For this review, take the finished solid that the model builds, in its own axes (mm). Give positions to 0.01 mm unless a question says otherwise; leave off trailing zeros. Order: outer loops, then holes, each group sorted by start corner. A loop starts at its lowest first (then second) coordinate and runs counter-clockwise, first axis right, second up. Notation, with made-up numbers: (-4.5, 31.5) -> (32.5, 31.5) arc R15 ccw to (32.5, 45.5) -> close; hole circle Ø7 at (68, 6). An arc over 180 degrees is marked (long way). Use CSV: the item, a comma, the result in double quotes. Start each with the question number.
Autodesk Inventor part; units mm, degrees
ref_plane "YZ Plane" through (0, 0, 0) normal (1, 0, 0) x (0, 1, 0)
ref_plane "XZ Plane" through (0, 0, 0) normal (0, 1, 0) x (-1, 0, 0)
ref_plane "XY Plane" through (0, 0, 0) normal (0, 0, 1) x (1, 0, 0)
sketch "Sketch1" plane through (0, 0, 0) normal (0, 1, 0) x (-1, 0, 0)
  line L0 (0, 0) -> (20.2618, 0)
  line L1 (20.2618, 0) -> (20.2618, -15.5601)
  line L2 (20.2618, -15.5601) -> (0, -15.5601)
  line L3 (0, -15.5601) -> (0, 0)
  dimension "d0" = 20.2618
  dimension "d1" = 15.5601
extrude "Extrusion1" add sketch "Sketch1" along normal blind 2.54
sketch "Sketch2" plane through (0, 2.54, 0) normal (0, 1, 0) x (1, 0, 0)
  circle A0 centre (-19.0703, 1.3447) radius 0.8937
  line L0 (-20.2618, 15.5601) -> (-20.2618, 0) construction
  line L1 (-20.2618, 0) -> (0, 0) construction
  line L2 (-20.2618, 0) -> (0, 0) construction
  circle A1 centre (-16.5303, 1.3447) radius 0.8937
  circle A2 centre (-13.9903, 1.3447) radius 0.8937
  circle A3 centre (-11.4503, 1.3447) radius 0.8937
  circle A4 centre (-8.9103, 1.3447) radius 0.8937
  circle A5 centre (-6.3703, 1.3447) radius 0.8937
  circle A6 centre (-3.8303, 1.3447) radius 0.8937
  circle A7 centre (-1.2903, 1.3447) radius 0.8937
  circle A8 centre (-17.7809, 13.0792) radius 1.5
  circle A9 centre (-2.4809, 13.0792) radius 1.5
  line L3 (0, 15.5601) -> (-20.2618, 15.5601)
  line L4 (0, 0) -> (0, 15.5601)
  line L5 (-17.7809, 13.0792) -> (-2.4809, 13.0792) construction
  line L6 (-10.1309, 0) -> (-10.1309, 15.5601) construction
  point P0 (-10.1309, 13.0792)
  dimension "d6" = 2.54
  dimension "d11" = 3
  dimension "d12" = 3
  dimension "d17" = 15.3
  dimension "d18" = 2.4809
  dimension "d19" = 2.4809
extrude "Extrusion2" cut sketch "Sketch2" against normal up to next
sketch "Sketch3" plane through (0, 2.54, 0) normal (0, 1, 0) x (1, 0, 0)
  line L0 (-14.6694, 9.1277) -> (-2.5672, 9.1277) construction
  line L1 (-2.5672, 9.1277) -> (-2.5672, 4.9306) construction
  line L2 (-2.5672, 4.9306) -> (-14.6694, 4.9306) construction
  line L3 (-14.6694, 4.9306) -> (-14.6694, 9.1277) construction
  point P0 (0, 0)
equation "\"d19\" = d18"
properties part number "IMU_temp"
1. Consider section C-C (z = -13.5). State the section outline as (x, y) points.
2. Consider section A-A (x = -9). State the section outline as (y, z) points, plus the area to 3 significant figures.
3. Consider section B-B (y = 0.4). State how many separate pieces and enclosed holes the cut face has, plus the area to 3 significant figures.
4. Draft analysis for pull direction X (two halves, no side actions). For faces 1 (the face through (-20.262, 1, -8)), 2 (the face through (0, 1, -8)), 3 (the face through (-10, 1, -15.56)), 4 (the face through (-15.705, 1.288, -1.002)), state which applies: +X half, -X half, draft (parallel to the pull), parting line (faces both ways), or undercut.
5. To check wall thickness, follow L1, parallel to X at y = 0.5, z = -13; L2, parallel to Z at x = -1.75, y = 0.65; L3, parallel to Z at x = -14, y = 0.3. State the ranges of each line that lie inside material, in increasing order. Write a range as [from, to].
6. Clearance check with a flat-ended pin moving along its axis: P1, Ø1.4, axis at x = -3.83, z = -1.34, coming from the +Y side. State where the tip first meets the part, or that it passes through.
7. Consider section D-D (x = -1.75). State the section outline as (y, z) points, plus the area to 3 significant figures.
Answer list:
1,outline,"(-20.26, 0) -> (-19.22, 0) -> (-19.22, 2.54) -> (-20.26, 2.54) -> close; (-16.34, 0) -> (-3.92, 0) -> (-3.92, 2.54) -> (-16.34, 2.54) -> close; (-1.04, 0) -> (0, 0) -> (0, 2.54) -> (-1.04, 2.54) -> close"
2,outline,"(0, -15.56) -> (2.54, -15.56) -> (2.54, -2.23) -> (0, -2.23) -> close; (0, -0.46) -> (2.54, -0.46) -> (2.54, 0) -> (0, 0) -> close"
2,area,"35.0 mm2"
3,separate pieces,"1"
3,enclosed holes,"10"
3,area,"281 mm2"
4,face 1,"-X half"
4,face 2,"+X half"
4,face 3,"draft"
4,face 4,"undercut"
5,L1,"[-20.26, -19.28], [-16.28, -3.98], [-0.98, 0]"
5,L2,"[-15.56, -14.39], [-11.77, -2.11], [-0.58, 0]"
5,L3,"[-15.56, -2.24], [-0.45, 0]"
6,P1,"through"
7,outline,"(0, -15.56) -> (2.54, -15.56) -> (2.54, -14.39) -> (0, -14.39) -> close; (0, -11.77) -> (2.54, -11.77) -> (2.54, -2.11) -> (0, -2.11) -> close; (0, -0.58) -> (2.54, -0.58) -> (2.54, 0) -> (0, 0) -> close"
7,area,"29.0 mm2"
